Geometry check sheet. Reference: the model listing, model coordinates, mm. A direction names the side the tool comes from. Round coordinates to 2 decimals unless told otherwise and drop trailing zeros. Loops run counter-clockwise (first coordinate to the right, second up) from the corner with the lowest first, then second, coordinate; pieces in that order, holes last. Notation, with made-up numbers: (41.5, 35.25) -> (52.5, 35.25) arc R25 ccw to (52.5, 61.25) -> close; hole circle Ø3 at (7, 26.25). An arc over 180 degrees is marked (long way). Use a Markdown table: item, result. Add a question column.
Q1. Gauge pin test, flat ends, axial feed: P1, Ø1, axis at x = 3.5, y = -3, coming from the +Z side; P2, Ø1, axis at y = -11.5, z = 0, coming from the +X side; P3, Ø1, axis at x = -4, y = -8.5, coming from the +Z side. Record the tip position at first contact, or that the pin passes through.
Q2. Set-up check for faces 1 (the face through (-2, -18.796, -4)), 2 (the face through (3.794, -9.905, 1.195)): record each of +Z, -Z, +X, -X, +Y, -Y from which the full face is reachable in a straight line by a thin tool's end or side.
Q3. Sectioned sample at B-B, the plane y = -1.75. Enter the section's corners in (x, z), then the cut area to 3 significant figures.
Q4. Release check for a two-part mould opening along X. For faces 3 (the face through (-3.76, -10.15, -2.89)), 4 (the face through (0, 0, 0)), 5 (the face through (0, -0.762, 0)) record: released by +X, released by -X, zero draft, split by the parting line, or undercut.
Q5. Material ranges on L1, parallel to Z at x = -2, y = -14.25; L2, parallel to Z at x = 0.5, y = -7; L3, parallel to X at y = -1.75, z = 2.75, recorded low to high.
Q6. Sectioned sample at A-A, the plane y = -8.75. Enter the section's corners in (x, z).
```python
from build123d import *

# Parameters (mm, degrees)
F0_R = 4.572
F2_R = 4.8895
F4_T = -0.762
F5_R = 1.27


with BuildPart() as f3:
    # F0 (on Front) → F3 section 0
    with BuildSketch(Plane.XZ):
        Circle(F0_R)
    # F2 (on offset) → F3 section 1
    with BuildSketch(Plane.XZ.offset(18.796)):
        Circle(F2_R)
    loft()

    # F4
    f4_openings = [f3.faces().sort_by_distance(p)[0] for p in [
        (0, -18.796, 0),
    ]]
    offset(amount=F4_T, openings=f4_openings, kind=Kind.INTERSECTION)

    # F5
    f5_edges = [f3.edges().sort_by_distance(p)[0] for p in [
        (-4.572, 0, 0),
    ]]
    fillet(f5_edges, radius=F5_R)


solid = f3.part
```
Values:
| question | item | result |
|---|---|---|
| 1 | P1 | z = 3.52 |
| 1 | P2 | x = 4.77 |
| 1 | P3 | z = 3.16 |
| 2 | face 1 | +Z, -Z, +X, -X, -Y |
| 2 | face 2 | -Y |
| 3 | outline | circle Ø9.2 at (0, 0); hole circle Ø7.68 at (0, 0) |
| 3 | area | 20.2 mm^2 |
| 4 | face 3 | split by the parting line |
| 4 | face 4 | zero draft |
| 4 | face 5 | undercut |
| 5 | L1 | -4.38 to -3.52, 3.52 to 4.38 |
| 5 | L2 | -4.66 to -3.9, 3.9 to 4.66 |
| 5 | L3 | -3.69 to -2.68, 2.68 to 3.69 |
| 6 | outline | circle Ø9.44 at (0, 0); hole circle Ø7.92 at (0, 0) |
